Read the model definition and answer for the solid it produces. Units are mm, in the model's axes. A direction names the side the tool comes from. Give positions to 0.01 mm unless a question says otherwise; leave off trailing zeros. Order: outer loops, then holes, each group sorted by start corner. A loop starts at its lowest first (then second) coordinate and runs counter-clockwise, first axis right, second up. Notation, with made-up numbers: M -35.75,85.5 L 15.25,85.5 A20 cw 15.25,116.5 Z; hole C -24,20.25 d11. An arc over 180 degrees is marked long. One line per item, written item: value.
from build123d import *

# Parameters (mm, degrees)
BOSS_EXTRUDE1_START      = -7
SKETCH1_R                = 2.5
SKETCH1_R_2              = 1.733910687
BOSS_EXTRUDE1_DEPTH      = 7
SKETCH2_R                = 1.688720836
BOSS_EXTRUDE2_DEPTH      = 200
BOSS_EXTRUDE2_DEPTH_BACK = 38.25
BOSS_EXTRUDE3_START      = 20
SKETCH3_R                = 7.5
BOSS_EXTRUDE3_DEPTH      = 30


with BuildPart() as part:
    # Sketch1 → Boss-Extrude1 (new body)
    with BuildSketch(Plane.XY.offset(166.922438479).offset(BOSS_EXTRUDE1_START)):
        with Locations((39.892028068, 76.700259913)):
            Circle(SKETCH1_R)
        with Locations((39.892028068, 76.700259913)):
            Circle(SKETCH1_R_2, mode=Mode.SUBTRACT)
    extrude(amount=-BOSS_EXTRUDE1_DEPTH)

    # Sketch2 → Boss-Extrude2 (add, two sides)
    with BuildSketch(Plane.XZ.offset(-36.700259913)) as boss_extrude2_sk:
        with Locations((39.892028068, 156.422438479)):
            Circle(SKETCH2_R)
    extrude(amount=BOSS_EXTRUDE2_DEPTH)
    extrude(boss_extrude2_sk.sketch, amount=-BOSS_EXTRUDE2_DEPTH_BACK)

    # Sketch3 → Boss-Extrude3 (add)
    with BuildSketch(Plane(origin=(0, -163.299740087, 0), x_dir=(-1, 0, 0), z_dir=(0, -1, 0)).offset(BOSS_EXTRUDE3_START)):
        with Locations((-39.892028068, -156.422438479)):
            Circle(SKETCH3_R)
    extrude(amount=-BOSS_EXTRUDE3_DEPTH)


solid = part.part
1) Find section B-B, the plane y = 59. Write down the section's boundary in (x, z), plus the area to 3 significant figures.
Reported:
outline: C 39.89,156.42 d3.38
area: 8.96 mm^2
2) Which of the six approach directions +Z, -Z, +X, -X, +Y, -Y give full straight-line access (tool end or side, diameter ignored) to faces 4 (the face through (39, 75, 159.922)), 5 (the face through (41.518, -168.51, 163.744))?
Reported:
face 4: +Z, +X, -X, +Y
face 5: +Y, -Y
3) Consider probe 1 along Y at (x, z) = (37.5, 160.5); probe 2 along Z at (x, y) = (39.5, 30.5); probe 3 along Z at (x, y) = (39.75, 65). Determine where each line is inside the solid, lowest interval first.
Reported:
probe 1: y = -183.3 to -153.3
probe 2: z = 154.78 to 158.07
probe 3: z = 154.74 to 158.11
4) Each of these flat-tipped pins is pushed along its axis until it touches: pin 1 Ø3 at (x, y) = (39.89, 76.7) entering from +Z; pin 2 Ø4.5 at (x, z) = (42.5, 155) entering from +Y; pin 3 Ø8 at (x, y) = (41, -66.5) entering from -Z; pin 4 Ø4 at (y, z) = (-123, 153) entering from +X. Where does it stop, or does it pass through?
Reported:
pin 1: passes through
pin 2: stops at y = 79.17
pin 3: stops at z = 154.73
pin 4: stops at x = 40.8
5) Determine the mould class of faces 1 (the face through (39.57, 79.18, 156.47)), 2 (the face through (40, -183.3, 156)), 3 (the face through (39, 75, 152.922)) for opening direction Y: +Y half, -Y half, draft (parallel to the pull), parting line (faces both ways), or undercut.
Reported:
face 1: undercut
face 2: -Y half
face 3: draft
6) Find section A-A, the plane y = -161.5. Write down the section's boundary in (x, z).
Reported:
outline: C 39.89,156.42 d15
